Model file for the job. Use its own axes, mm. Face numbers are marked on the shaded views. A direction names the side the tool comes from. Round coordinates to 2 decimals unless told otherwise and drop trailing zeros. Write each loop counter-clockwise with the first axis right and the second up, starting at its lowest first coordinate (ties: lowest second). Pieces come first, ordered by that corner, then holes.
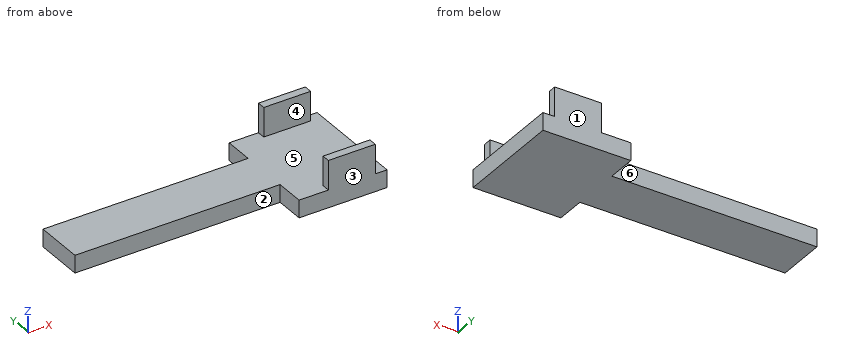
```python
from build123d import *

# Parameters (mm, degrees)
SKETCH2_W           = 63.5
SKETCH2_H           = 23.368
BOSS_EXTRUDE1_DEPTH = 3.81
SKETCH3_W           = 12.7
SKETCH3_H           = 1.778
BOSS_EXTRUDE2_DEPTH = 6.35
SKETCH4_W           = 2.54
SKETCH4_H           = 6.35
CUT_EXTRUDE1_DEPTH  = 24.368
SKETCH5_W           = 44.45
SKETCH5_H           = 6.35
CUT_EXTRUDE2_DEPTH  = 4.81
SCALE1_SCALE        = 1.02


with BuildPart() as part:
    # Sketch2 → Boss-Extrude1 (new body)
    with BuildSketch(Plane.XY):
        Rectangle(SKETCH2_W, SKETCH2_H)
    extrude(amount=BOSS_EXTRUDE1_DEPTH)

    # Sketch3 → Boss-Extrude2 (add)
    with BuildSketch(Plane.XY.offset(3.81)):
        with Locations((25.4, 10.795)):
            Rectangle(SKETCH3_W, SKETCH3_H)
        with Locations((25.4, -10.795)):
            Rectangle(SKETCH3_W, SKETCH3_H)
    extrude(amount=BOSS_EXTRUDE2_DEPTH)

    # Sketch4 → Cut-Extrude1 (cut, through all)
    with BuildSketch(Plane(origin=(0, 11.684, 0), x_dir=(1, 0, 0), z_dir=(0, 1, 0))):
        with Locations((30.48, -6.985)):
            Rectangle(SKETCH4_W, SKETCH4_H)
    extrude(amount=-CUT_EXTRUDE1_DEPTH, mode=Mode.SUBTRACT)

    # Sketch5 → Cut-Extrude2 (cut, through all)
    with BuildSketch(Plane.XY.offset(3.81)):
        with Locations((-9.525, -8.509)):
            Rectangle(SKETCH5_W, SKETCH5_H)
    cut_extrude2 = extrude(amount=-CUT_EXTRUDE2_DEPTH, mode=Mode.SUBTRACT)

    # Mirror1: Cut-Extrude2 across plane
    add(cut_extrude2.mirror(Plane.ZX), mode=Mode.SUBTRACT)


with BuildPart() as part_1:
    # Scale1: scaled about (6.972453348, 0, 2.217272228)
    add(part.part.scale(SCALE1_SCALE).moved(Location((-0.139449067, 0, -0.044345445))))


solid = part_1.part
```
1) Flat gauge pins, fed straight in: pin 1 Ø1.2 at (x, z) = (-13, 1) entering from +Y; pin 2 Ø4.5 at (x, z) = (-1, 2) entering from -Y; pin 3 Ø4.5 at (y, z) = (-8.5, 1) entering from -X. Where does each tip first touch, or does it go through?
2) Which spindle directions (+Z, -Z, +X, -X, +Y, -Y) get a long thin tool onto all of the face, cutting with end or side? Do the marked faces 1 and 2. Say none if no direction does.
3) Pull direction Y, two halves, no side cores. Call the marked faces 3, 4, 5 and 6: released by +Y, released by -Y, zero draft, split by the parting line, or undercut.
4) Cut at C-C on x = -25. List the corners of the cut face in (y, z), and give its area (3 significant figures).
5) Cut at D-D on z = 1.5. List the corners of the cut face in (x, y).
6) Wall check: probe 1 along Y at (x, z) = (27, 7.75); probe 2 along Z at (x, y) = (24.5, -7.5); probe 3 along X at (y, z) = (6.75, 2.75). Give the ranges that are in metal, low to high.
7) Cut at A-A on z = 6.75. List the corners of the cut face in (x, y).
8) Cut at B-B on y = 0. List the corners of the cut face in (x, z), and give its area (3 significant figures).
Result sheet:
1. pin 1: stops at y = 5.44
1. pin 2: stops at y = -5.44
1. pin 3: stops at x = 12.81
2. face 1: +Z, -Z, +X, -X, +Y
2. face 2: +Z, -Z, -X, -Y
3. face 3: released by -Y
3. face 4: undercut
3. face 5: undercut
3. face 6: released by +Y
4. outline: (-5.44, -0.04) - (5.44, -0.04) - (5.44, 3.84) - (-5.44, 3.84) - close
4. area: 42.3 mm2
5. outline: (-32.52, -5.44) - (12.81, -5.44) - (12.81, -11.92) - (32.25, -11.92) - (32.25, 11.92) - (12.81, 11.92) - (12.81, 5.44) - (-32.52, 5.44) - close
6. probe 1: y = -11.92 to -10.1, 10.1 to 11.92
6. probe 2: z = -0.04 to 3.84
6. probe 3: x = 12.81 to 32.25
7. outline: (19.29, -11.92) - (29.65, -11.92) - (29.65, -10.1) - (19.29, -10.1) - close; (19.29, 10.1) - (29.65, 10.1) - (29.65, 11.92) - (19.29, 11.92) - close
8. outline: (-32.52, -0.04) - (32.25, -0.04) - (32.25, 3.84) - (-32.52, 3.84) - close
8. area: 252 mm2
